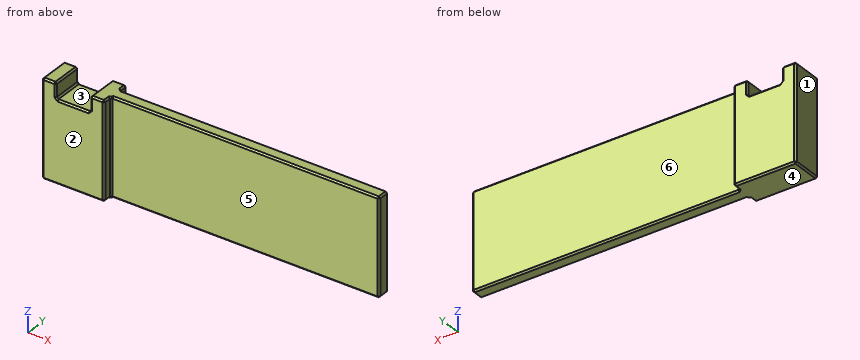
```python
from build123d import *

# Parameters (mm, degrees)
SKETCH1_W           = 106
SKETCH1_H           = 31
BOSS_EXTRUDE1_DEPTH = 4
SKETCH2_W           = 20
SKETCH2_H           = 31
BOSS_EXTRUDE2_DEPTH = 5
SKETCH3_W           = 11
SKETCH3_H           = 5
CUT_EXTRUDE1_DEPTH  = 11
CHAMFER1_SIZE       = 0.5


with BuildPart() as part:
    # Sketch1 → Boss-Extrude1 (new body)
    with BuildSketch(Plane(origin=(0, 0, 0), x_dir=(1, 0, 0), z_dir=(0, 1, 0))):
        with Locations((53, 15.5)):
            Rectangle(SKETCH1_W, SKETCH1_H)
    extrude(amount=BOSS_EXTRUDE1_DEPTH)

    # Sketch2 → Boss-Extrude2 (add, symmetric)
    with BuildSketch(Plane(origin=(0, 2, 0), x_dir=(1, 0, 0), z_dir=(0, 1, 0))):
        with Locations((10, 15.5)):
            Rectangle(SKETCH2_W, SKETCH2_H)
    extrude(amount=BOSS_EXTRUDE2_DEPTH, both=True)

    # Sketch3 → Cut-Extrude1 (cut, through all)
    with BuildSketch(Plane(origin=(0, 7, 0), x_dir=(1, 0, 0), z_dir=(0, 1, 0))):
        with Locations((10, 2.5)):
            Rectangle(SKETCH3_W, SKETCH3_H)
    extrude(amount=-CUT_EXTRUDE1_DEPTH, mode=Mode.SUBTRACT)

    # Chamfer1
    chamfer1_edges = [part.edges().sort_by_distance(p)[0] for p in [
        (106, 4, -15.5),
        (63, 0, 0),
        (20, 0, -15.5),
        (63, 4, 0),
        (63, 4, -31),
        (20, 5.5, 0),
        (20, 4, -15.5),
        (20, 5.5, -31),
        (0, -3, -15.5),
        (2.25, -3, 0),
        (20, -1.5, 0),
        (20, -3, -15.5),
        (20, -1.5, -31),
        (10, -3, -31),
        (0, 7, -15.5),
        (2.25, 7, 0),
        (20, 7, -15.5),
        (10, 7, -31),
        (17.75, 7, 0),
        (17.75, -3, 0),
        (4.5, -3, -2.5),
        (4.5, 2, 0),
        (10, -3, -5),
        (4.5, 2, -5),
        (15.5, -3, -2.5),
        (15.5, 2, -5),
        (15.5, 2, 0),
        (4.5, 7, -2.5),
        (15.5, 7, -2.5),
        (10, 7, -5),
        (63, 0, -31),
        (106, 0, -15.5),
        (0, 2, -31),
        (106, 2, -31),
        (106, 2, 0),
        (0, 2, 0),
    ]]
    chamfer(chamfer1_edges, length=CHAMFER1_SIZE)


solid = part.part
```
Geometry check sheet. Reference: the model listing, model coordinates, mm. Face numbers are marked on the shaded views. A direction names the side the tool comes from. Round coordinates to 2 decimals unless told otherwise and drop trailing zeros. Order: outer loops, then holes, each group sorted by start corner. A loop starts at its lowest first (then second) coordinate and runs counter-clockwise, first axis right, second up. Notation, with made-up numbers: (-14, -2) - (16, -2) arc R31 ccw to (16, 31) - close; hole circle Ø10 at (0.25, 29.5). An arc over 180 degrees is marked (long way). Use a Markdown table: item, result. Add a question column.
(1) Sectioned sample at B-B, the plane y = -1.5. Enter the section's corners in (x, z).
(2) Release check for a two-part mould opening along X. For the marked faces 1, 2 and 3 record: pulls with the +X half, pulls with the -X half, needs draft (parallel to the pull), parting line crosses it, or undercut.
(3) Material ranges on line 1 along Y through (x, z) = (71.5, -8); line 2 along X through (y, z) = (-1.5, -12.5); line 3 along X through (y, z) = (4.25, -3.5), recorded low to high. Write a range as [from, to].
(4) Sectioned sample at C-C, the plane x = 40.5. Enter the section's corners in (y, z).
(5) Depth check by flat-ended pin: pin 1 (1 mm diameter, centred on y = 6, z = -19, fed in from +X); pin 2 (9 mm diameter, centred on x = 56, z = -10, fed in from +Y); pin 3 (2.5 mm diameter, centred on x = 10.5, y = 2.5, fed in from +Z). Enter the tip coordinate at first touch or a pass-through.
(6) Tool access check on the marked faces 4, 5 and 6. Record the directions out of +Z, -Z, +X, -X, +Y, -Y that give a thin tool (end or side, any length) a straight path to the whole face; none if there is none.
(7) Sectioned sample at A-A, the plane z = -9.5. Enter the section's corners in (x, y), and give its area (4 significant figures).
Answers below:
| question | item | result |
|---|---|---|
| 1 | outline | (0, -30.5) - (0.5, -31) - (19.5, -31) - (20, -30.5) - (20, -0.5) - (19.5, 0) - (16, 0) - (15.5, -0.5) - (15.5, -4.5) - (15, -5) - (5, -5) - (4.5, -4.5) - (4.5, -0.5) - (4, 0) - (0.5, 0) - (0, -0.5) - close |
| 2 | face 1 | pulls with the -X half |
| 2 | face 2 | needs draft |
| 2 | face 3 | undercut |
| 3 | line 1 | [0, 4] |
| 3 | line 2 | [0, 20] |
| 3 | line 3 | [0, 4.5], [15.5, 20.25] |
| 4 | outline | (0, -30.5) - (0.5, -31) - (3.5, -31) - (4, -30.5) - (4, -0.5) - (3.5, 0) - (0.5, 0) - (0, -0.5) - close |
| 5 | pin 1 | x = 20 |
| 5 | pin 2 | y = 4 |
| 5 | pin 3 | z = -5 |
| 6 | face 4 | -Z, +X, -X, +Y, -Y |
| 6 | face 5 | +Z, -Z, +X, -Y |
| 6 | face 6 | +Z, -Z, +X, +Y |
| 7 | outline | (0, -2.5) - (0.5, -3) - (19.5, -3) - (20, -2.5) - (20, -0.5) - (20.5, 0) - (105.5, 0) - (106, 0.5) - (106, 3.5) - (105.5, 4) - (20.5, 4) - (20, 4.5) - (20, 6.5) - (19.5, 7) - (0.5, 7) - (0, 6.5) - close |
| 7 | area | 543.5 mm² |
